from build123d import *

# Parameters (mm, degrees)
SKETCH1_R           = 1
BOSS_EXTRUDE1_DEPTH = 8
CUT_EXTRUDE1_START  = 9.5
CUT_EXTRUDE1_DEPTH  = 1.1


with BuildPart() as part:
    # Sketch1 → Boss-Extrude1 (new body)
    with BuildSketch(Plane(origin=(0, 0, 0), x_dir=(1, 0, 0), z_dir=(0, 1, 0))):
        with Locations(Location((0, 0, 0), (0, 0, 270))):
            Circle(SKETCH1_R)
    extrude(amount=BOSS_EXTRUDE1_DEPTH)

    # Sketch2 → Revolve2 (revolve)
    with BuildSketch(Plane.XY, mode=Mode.PRIVATE) as revolve2_sk:
        with BuildLine():
            Line((0, 8), (-2, 8))
            Line((-2, 8), (-2, 8.5))
            ThreePointArc((-2, 8.5), (-1.055436608, 9.001787176), (0, 9.17511905))
            Line((0, 9.17511905), (0, 8))
        make_face()
    revolve(revolve2_sk.sketch.rotate(Axis((0, 8, 0), (0, 1, 0)), 180), axis=Axis((0, 8, 0), (0, 1, 0)))

    # Sketch3 → Cut-Extrude1 (cut)
    with BuildSketch(Plane(origin=(0, 0, 0), x_dir=(1, 0, 0), z_dir=(0, 1, 0)).offset(CUT_EXTRUDE1_START)):
        Polygon((0.433012702, -0.75), (0.866025404, 0), (0.433012702, 0.75), (-0.433012702, 0.75), (-0.866025404, 0), (-0.433012702, -0.75), align=None)
    extrude(amount=-CUT_EXTRUDE1_DEPTH, mode=Mode.SUBTRACT)


solid = part.part
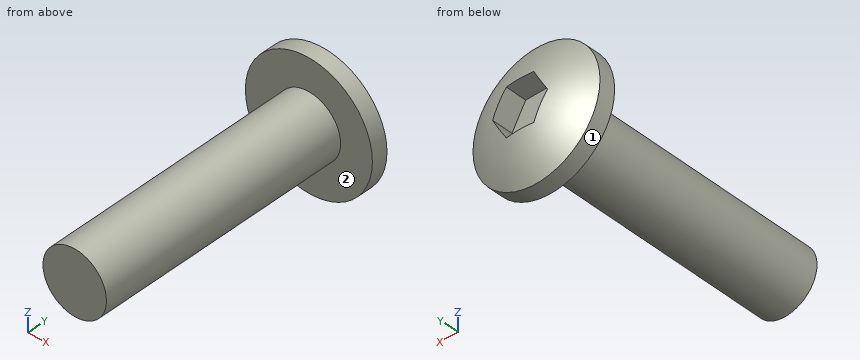
Model file for the job. Use its own axes, mm. Face numbers are marked on the shaded views. A direction names the side the tool comes from. Give positions to 0.01 mm unless a question says otherwise; leave off trailing zeros. Loops run counter-clockwise (first coordinate to the right, second up) from the corner with the lowest first, then second, coordinate; pieces in that order, holes last.
1) Saw through at B-B (y = 1.75). Write the cut outline in (x, z).
2) Saw through at C-C (z = -0.55). Write the cut outline in (x, y).
3) Flat gauge pins, fed straight in: pin 1 Ø1 at (x, y) = (-1, 6) entering from -Z; pin 2 Ø1.5 at (x, y) = (0.5, 1.5) entering from +Z. Where does each tip first touch, or does it go through?
4) Wall check: line 1 (X direction, y = 2.25, z = -0.05); line 2 (Y direction, x = -0.95, z = 1.05); line 3 (Y direction, x = 0.55, z = 1.35). Give the ranges that are in metal, low to high.
5) Tool access for the marked faces 1 and 2: list every direction of +Z, -Z, +X, -X, +Y, -Y with a clear straight run to the whole face (end or side of a thin tool).
6) Saw through at A-A (x = 0). Write the cut outline in (y, z), plus the area to 3 significant figures.
7) Saw through at D-D (x = -1.7). Write the cut outline in (y, z), plus the area to 3 significant figures.
Answer block:
1. outline: circle Ø2 at (0, 0)
2. outline: (-1.92, 8) - (-0.84, 8) - (-0.84, 0) - (0.84, 0) - (0.84, 8) - (1.92, 8) - (1.92, 8.5) arc R3.25 ccw to (0.55, 9.08) - (0.55, 8.4) - (-0.55, 8.4) - (-0.55, 9.08) arc R3.25 ccw to (-1.92, 8.5) - close
3. pin 1: stops at z = -0.87
3. pin 2: stops at z = 1
4. line 1: x = -1 to 1
4. line 2: y = 8 to 8.86
4. line 3: y = 8 to 8.84
5. face 1: +Y, -Y
5. face 2: -Y
6. outline: (0, -1) - (8, -1) - (8, -2) - (8.5, -2) arc R3.3 ccw to (9.09, -0.75) - (8.4, -0.75) - (8.4, 0.75) - (9.09, 0.75) arc R3.3 ccw to (8.5, 2) - (8, 2) - (8, 1) - (0, 1) - close
6. area: 18.7 mm2
7. outline: (8, -1.05) - (8.5, -1.05) arc R2.83 ccw to (8.5, 1.05) - (8, 1.05) - close
7. area: 1.34 mm2
